Verification items for this drawing (mm, ordinates from the low corner). Round coordinates to 2 decimals unless told otherwise and drop trailing zeros. Order: outer loops, then holes, each group sorted by start corner. A loop starts at its lowest first (then second) coordinate and runs counter-clockwise, first axis right, second up. Notation, with made-up numbers: M 24,-5.75 L 64,-5.75 A16 ccw 64,0.25 Z; hole C 47.5,85.25 d8. An arc over 180 degrees is marked long. One line per item, written item: value. Start each with the question number.
(1) Cross-section at A-A, the plane z = 40. Enter the section's corners in (x, y).
(2) Thickness scan on L1, parallel to Z at x = 25, y = 1.15; L2, parallel to Z at x = 25.5, y = 1.5 (1 decimal); L3, parallel to X at y = 1.95, z = 10.5. Record the ranges inside material, lowest first.
(3) Cross-section at B-B, the plane z = 25. Enter the section's corners in (x, y), and give its area (3 significant figures).
(4) Depth check by flat-ended pin: pin 1 Ø2 at (x, y) = (18, 1) entering from +Z; pin 2 Ø4 at (x, z) = (45, 25) entering from -Y. Enter the tip coordinate at first touch or a pass-through.
(5) Cross-section at D-D, the plane x = 19.5. Enter the section's corners in (y, z).
(6) Cross-section at C-C, the plane x = 5. Enter the section's corners in (y, z).
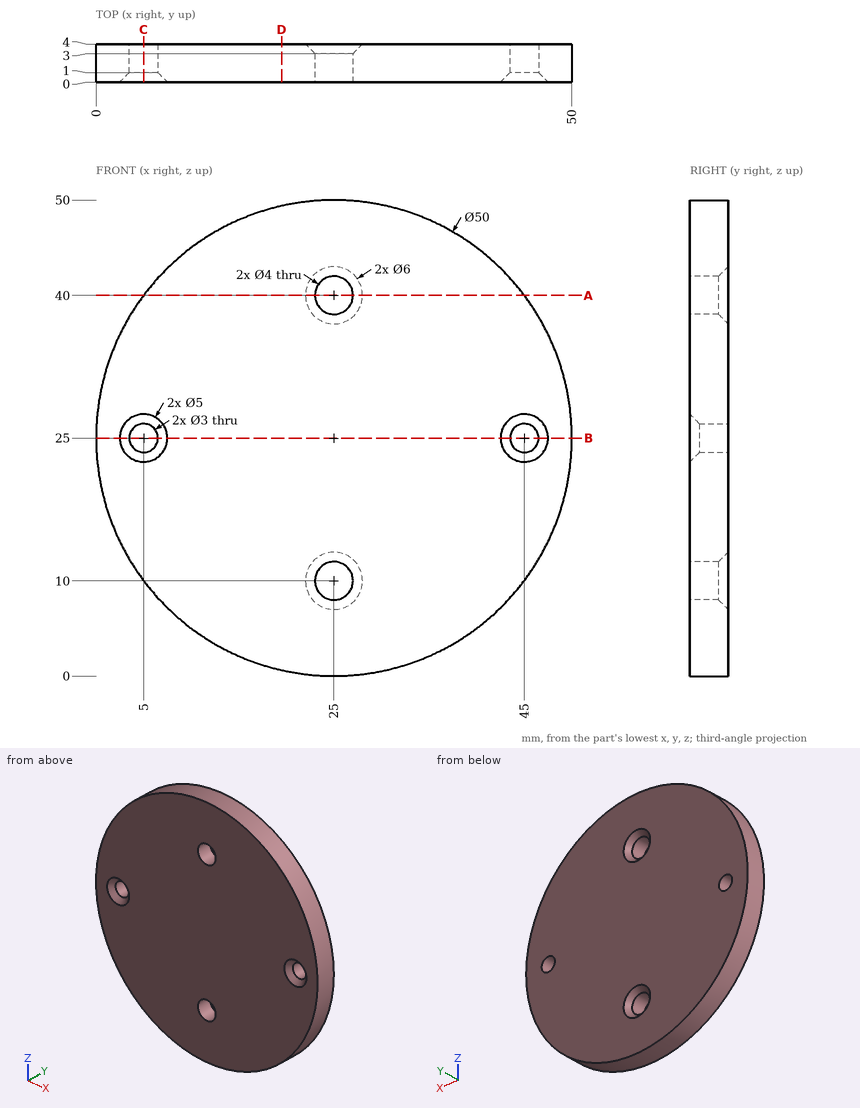
Values found:
1. outline: M 5,0 L 23,0 L 23,3 L 22,4 L 5,4 Z; M 27,0 L 45,0 L 45,4 L 28,4 L 27,3 Z
2. L1: 0 to 8, 12 to 38, 42 to 50
2. L2: 0 to 8.1, 11.9 to 38.1, 41.9 to 50
2. L3: 4.63 to 23.06, 26.94 to 45.37
3. outline: M 0,0 L 2.5,0 L 3.5,1 L 3.5,4 L 0,4 Z; M 6.5,1 L 7.5,0 L 42.5,0 L 43.5,1 L 43.5,4 L 6.5,4 Z; M 46.5,1 L 47.5,0 L 50,0 L 50,4 L 46.5,4 Z
3. area: 174 mm^2
4. pin 1: z = 49.27
4. pin 2: y = 0.5
5. outline: M 0,0.61 L 4,0.61 L 4,49.39 L 0,49.39 Z
6. outline: M 0,10 L 4,10 L 4,23.5 L 1,23.5 L 0,22.5 Z; M 0,27.5 L 1,26.5 L 4,26.5 L 4,40 L 0,40 Z
